Part model, mm, in its own coordinate system. A direction names the side the tool comes from. Give positions to 0.01 mm unless a question says otherwise; leave off trailing zeros. Loops run counter-clockwise (first coordinate to the right, second up) from the corner with the lowest first, then second, coordinate; pieces in that order, holes last. Notation, with made-up numbers: M 81,19.25 L 85,19.25 A23 cw 85,54.25 Z; hole C 79.25,-3.75 d6. An arc over 180 degrees is marked long. Answer in a Markdown table with one row per item.
from build123d import *

# Parameters (mm, degrees)
SKETCH1_R           = 35
SKETCH1_R_2         = 25
BOSS_EXTRUDE1_DEPTH = 50
BOSS_EXTRUDE2_DEPTH = 16


with BuildPart() as part:
    # Sketch1 → Boss-Extrude1 (new body)
    with BuildSketch(Plane(origin=(0, 0, 0), x_dir=(0, 1, 0), z_dir=(0, 0, 1))):
        with Locations(Location((0, 0, 0), (0, 0, 270))):
            Circle(SKETCH1_R)
        with Locations(Location((0, 0, 0), (0, 0, 270))):
            Circle(SKETCH1_R_2, mode=Mode.SUBTRACT)
    extrude(amount=BOSS_EXTRUDE1_DEPTH)

    # Sketch1_3 → Boss-Extrude2 (add)
    with BuildSketch(Plane(origin=(0, 0, 0), x_dir=(0, 1, 0), z_dir=(0, 0, 1))):
        with BuildLine():
            Line((75, 25), (24.494897428, 25))
            ThreePointArc((24.494897428, 25), (29.971518449, 18.075067963), (33.541019662, 10))
            Line((33.541019662, 10), (75, 10))
            Line((75, 10), (75, 25))
        make_face()
        with BuildLine():
            ThreePointArc((33.541019662, -10), (29.971518449, -18.075067963), (24.494897428, -25))
            Line((24.494897428, -25), (75, -25))
            Line((75, -25), (75, -10))
            Line((75, -10), (33.541019662, -10))
        make_face()
        with BuildLine():
            Line((-33.541019662, -10), (-75, -10))
            Line((-75, -10), (-75, -25))
            Line((-75, -25), (-24.494897428, -25))
            ThreePointArc((-24.494897428, -25), (-29.971518449, -18.075067963), (-33.541019662, -10))
        make_face()
        with BuildLine():
            Line((-75, 10), (-33.541019662, 10))
            ThreePointArc((-33.541019662, 10), (-29.971518449, 18.075067963), (-24.494897428, 25))
            Line((-24.494897428, 25), (-75, 25))
            Line((-75, 25), (-75, 10))
        make_face()
    extrude(amount=BOSS_EXTRUDE2_DEPTH)


solid = part.part
(1) Drill centre lines: line 1 along X through (y, z) = (-0.5, 19) (3 decimals); line 2 along Y through (x, z) = (0, 14); line 3 along Z through (x, y) = (15.5, 60). Where is each one in solid material? Low to high.
Recorded:
| item | result |
|---|---|
| line 1 | x = -34.996 to -24.995, 24.995 to 34.996 |
| line 2 | y = -35 to -25, 25 to 35 |
| line 3 | z = 0 to 16 |
(2) Which spindle directions (+Z, -Z, +X, -X, +Y, -Y) get a long thin tool onto all of the face, cutting with end or side? Do faces 1 (the face through (-25, 50, 8)), 2 (the face through (-25, -49, 8)), 3 (the face through (25, 49, 8)), 4 (the face through (-18, 49, 16)). Say none if no direction does.
Recorded:
| item | result |
|---|---|
| face 1 | +Z, -Z, -X, +Y |
| face 2 | +Z, -Z, -X, -Y |
| face 3 | +Z, -Z, +X, +Y |
| face 4 | +Z, -X, +Y |
(3) Saw through at A-A (y = 0). Write the cut outline in (x, z), plus the area to 3 significant figures.
Recorded:
| item | result |
|---|---|
| outline | M -35,0 L -25,0 L -25,50 L -35,50 Z; M 25,0 L 35,0 L 35,50 L 25,50 Z |
| area | 1,000 mm^2 |
(4) Saw through at C-C (z = 8.5). Write the cut outline in (x, y), plus the area to 3 significant figures.
Recorded:
| item | result |
|---|---|
| outline | M -25,-75 L -10,-75 L -10,-33.54 A35 ccw 10,-33.54 L 10,-75 L 25,-75 L 25,-24.49 A35 ccw 25,24.49 L 25,75 L 10,75 L 10,33.54 A35 ccw -10,33.54 L -10,75 L -25,75 L -25,24.49 A35 ccw -25,-24.49 Z; hole C 0,0 d50 |
| area | 4,590 mm^2 |
(5) Pin check, flat tips, straight feed: pin 1 Ø13 at (y, z) = (57, 4.5) entering from +X; pin 2 Ø12 at (x, y) = (20.5, -52) entering from +Z; pin 3 Ø1 at (y, z) = (-27.5, 17) entering from +X. Stop position of each tip, or through.
Recorded:
| item | result |
|---|---|
| pin 1 | stops at x = 25 |
| pin 2 | stops at z = 16 |
| pin 3 | stops at x = 22.27 |
(6) Pull direction X, two halves, no side cores. Call faces 5 (the face through (10, 55, 8)), 6 (the face through (25, -50, 8)), 7 (the face through (-10, -55, 8)), 8 (the face through (17, -75, 8)): +X half, -X half, draft (parallel to the pull), parting line (faces both ways), or undercut.
Recorded:
| item | result |
|---|---|
| face 5 | undercut |
| face 6 | +X half |
| face 7 | undercut |
| face 8 | draft |
(7) Saw through at D-D (x = 15). Write the cut outline in (y, z), plus the area to 3 significant figures.
Recorded:
| item | result |
|---|---|
| outline | M -75,0 L -20,0 L -20,50 L -31.62,50 L -31.62,16 L -75,16 Z; M 20,0 L 75,0 L 75,16 L 31.62,16 L 31.62,50 L 20,50 Z |
| area | 2,550 mm^2 |
